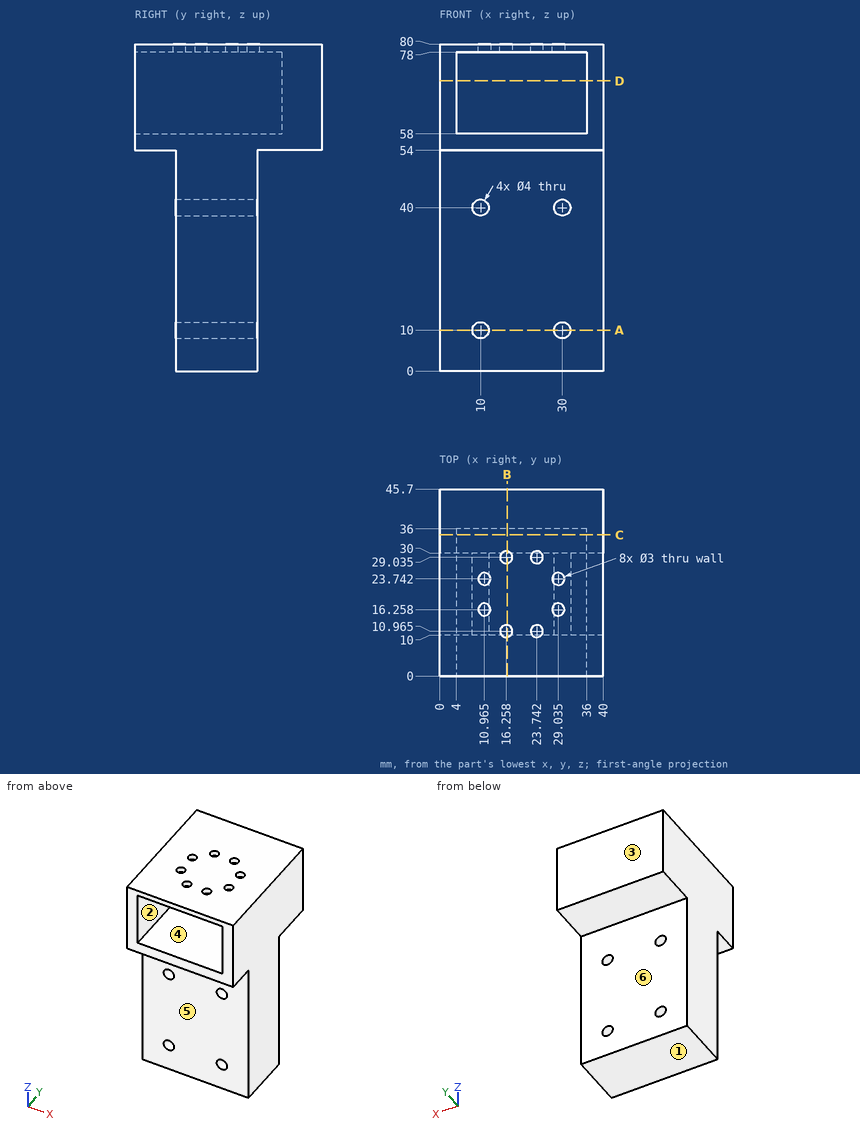
Could you check a few things on this drawing? It's one solid part, dimensions in mm from its lowest x, y, z. A direction names the side the tool comes from. Round coordinates to 2 decimals unless told otherwise and drop trailing zeros. Write each loop counter-clockwise with the first axis right and the second up, starting at its lowest first coordinate (ties: lowest second). Pieces come first, ordered by that corner, then holes. Notation, with made-up numbers: (77.25, 66) -> (112.25, 66) arc R16 cw to (112.25, 72) -> close; hole circle Ø4 at (-8, 25.5). An arc over 180 degrees is marked (long way). One line per question, with ' | ' between items. Start each with the question number.
1) If we mould it in two halves opening along Z, with no side actions, what happens to the marked faces 1, 2 and 3? For each: released by +Z, released by -Z, zero draft, split by the parting line, or undercut.
2) I need wall thicknesses on line 1 (Z direction, x = 13.5, y = 35); line 2 (Z direction, x = 13, y = 12); line 3 (Z direction, x = 30, y = 20.75). Which ranges of each line are inside material? Lowest first, please. Write a range as [from, to].
3) On a 3-axis mill with a long thin cutter (end or side, diameter ignored), from which of +Z, -Z, +X, -X, +Y, -Y can I reach the whole of each face in a straight line? I mean the marked faces 4, 5 and 6. Say none if no direction works.
4) Suppose I cut it at A-A on z = 10. Write out the boundary of the cut face in (x, y), then the cut area to 3 significant figures.
5) Suppose I cut it at C-C on y = 34.5. Write out the boundary of the cut face in (x, z), then the cut area to 3 significant figures.
6) Suppose I cut it at D-D on z = 71. Write out the boundary of the cut face in (x, y), then the cut area to 3 significant figures.
7) Suppose I cut it at B-B on x = 16.5. Write out the boundary of the cut face in (y, z) (1 decimal), then the cut area to 3 significant figures.
8) I'm going to push flat-ended pins straight in: P1, Ø4, axis at x = 14, y = 36, coming from the -Z side; P2, Ø16, axis at x = 25.5, z = 69, coming from the -Y side; P3, Ø6, axis at x = 12.5, z = 37, coming from the +Y side. Where does each tip first touch, or does it pass through?
Return value:
1) face 1: released by -Z | face 2: undercut | face 3: zero draft
2) line 1: z = [54, 58], [78, 80] | line 2: z = [0, 58], [78, 80] | line 3: z = [0, 8], [12, 38], [42, 58], [78, 80]
3) face 4: -Y | face 5: -Z, +X, -X, -Y | face 6: -Z, +X, -X, +Y
4) outline: (0, 10) -> (8, 10) -> (8, 30) -> (0, 30) -> close; (12, 10) -> (28, 10) -> (28, 30) -> (12, 30) -> close; (32, 10) -> (40, 10) -> (40, 30) -> (32, 30) -> close | area: 640 mm2
5) outline: (0, 54) -> (40, 54) -> (40, 80) -> (0, 80) -> close; hole (4, 58) -> (36, 58) -> (36, 78) -> (4, 78) -> close | area: 400 mm2
6) outline: (0, 0) -> (4, 0) -> (4, 36) -> (36, 36) -> (36, 0) -> (40, 0) -> (40, 45.7) -> (0, 45.7) -> close | area: 676 mm2
7) outline: (0, 54) -> (10, 54) -> (10, 0) -> (30, 0) -> (30, 54) -> (45.7, 54) -> (45.7, 80) -> (30.5, 80) -> (30.5, 78) -> (36, 78) -> (36, 58) -> (0, 58) -> close; (0, 78) -> (9.5, 78) -> (9.5, 80) -> (0, 80) -> close; (12.4, 78) -> (27.6, 78) -> (27.6, 80) -> (12.4, 80) -> close | area: 1,540 mm2
8) P1: stops at z = 54 | P2: stops at y = 36 | P3: stops at y = 30
